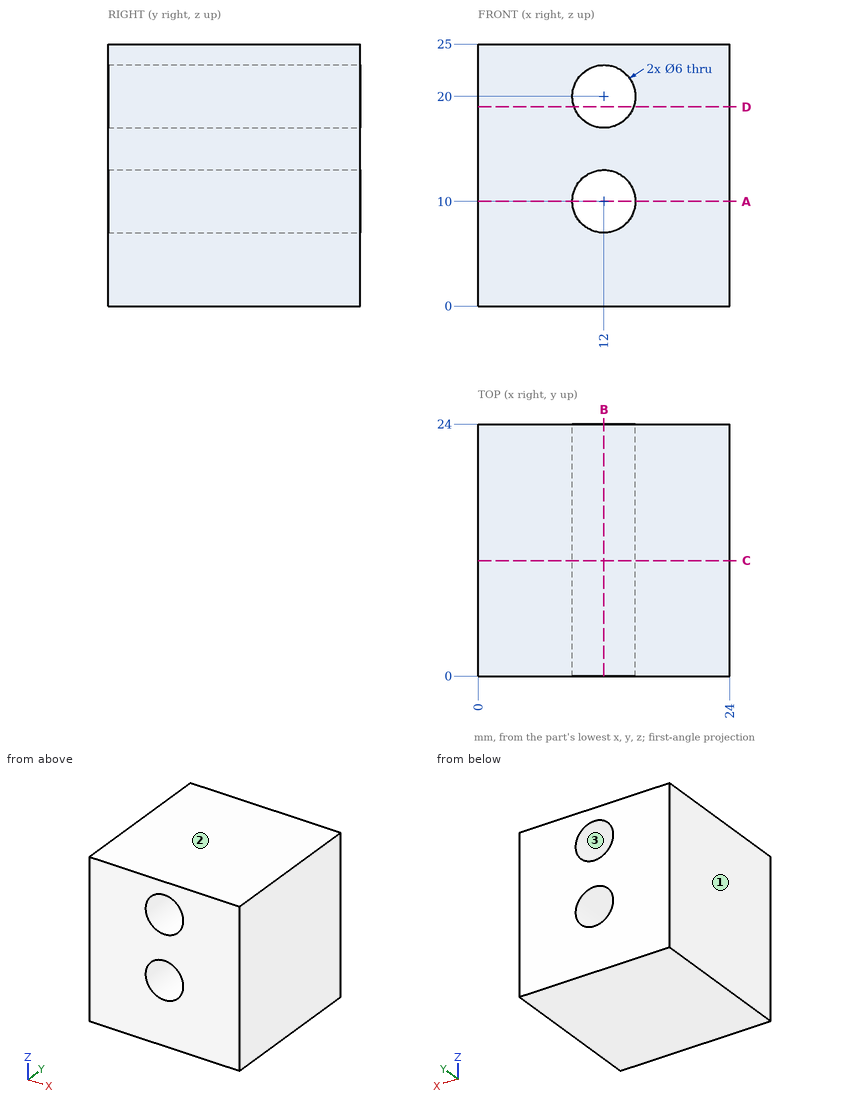
Geometry: see drawing. Coordinates: mm, zero at the bounding-box minimum. Give positions to 0.01 mm unless a question says otherwise; leave off trailing zeros. Write each loop counter-clockwise with the first axis right and the second up, starting at its lowest first coordinate (ties: lowest second). Pieces come first, ordered by that corner, then holes. Notation, with made-up numbers: M 26.25,-3 L 48.25,-3 A14 ccw 48.25,24 Z; hole C 3,89 d3. An arc over 180 degrees is marked long. Answer in a Markdown table with one row per item. Add a question column.
(1) Section C-C on y = 11. Return loops of the section in (x, z).
(2) Ray query, line 1 (Z direction, x = 12, y = 10.25); line 2 (X direction, y = 19.5, z = 10.25); line 3 (X direction, y = 15.75, z = 8.5). Return the intervals inside material, ascending.
(3) Section B-B on x = 12. Return loops of the section in (y, z).
(4) Section D-D on z = 19. Return loops of the section in (x, y), and give its area (3 significant figures).
(5) First-contact query: pin 1 (1.5 mm diameter, centred on x = 12.5, z = 17, fed in from -Y); pin 2 (5.5 mm diameter, centred on x = 12, z = 20, fed in from +Y). Flat tips, straight axial feed; report the tip coordinate or a pass-through.
(6) Section A-A on z = 10. Return loops of the section in (x, y).
(7) Mould query, pull axis X, two halves, no side actions, for the marked faces 1, 2 and 3. Classes: +X half, -X half, draft (parallel to the pull), parting line (faces both ways), or undercut.
Result set:
| question | item | result |
|---|---|---|
| 1 | outline | M 0,0 L 24,0 L 24,25 L 0,25 Z; hole C 12,10 d6; hole C 12,20 d6 |
| 2 | line 1 | z = 0 to 7, 13 to 17, 23 to 25 |
| 2 | line 2 | x = 0 to 9.01, 14.99 to 24 |
| 2 | line 3 | x = 0 to 9.4, 14.6 to 24 |
| 3 | outline | M 0,0 L 24,0 L 24,7 L 0,7 Z; M 0,13 L 24,13 L 24,17 L 0,17 Z; M 0,23 L 24,23 L 24,25 L 0,25 Z |
| 4 | outline | M 0,0 L 9.17,0 L 9.17,24 L 0,24 Z; M 14.83,0 L 24,0 L 24,24 L 14.83,24 Z |
| 4 | area | 440 mm^2 |
| 5 | pin 1 | stops at y = 0 |
| 5 | pin 2 | passes through |
| 6 | outline | M 0,0 L 9,0 L 9,24 L 0,24 Z; M 15,0 L 24,0 L 24,24 L 15,24 Z |
| 7 | face 1 | -X half |
| 7 | face 2 | draft |
| 7 | face 3 | undercut |
